```python
from build123d import *

# Parameters (mm, degrees)
F0_W     = 20
F0_H     = 95
F1_DEPTH = 6
F3_R     = 3
F5_R     = 4.25
F5_R_2   = 3
F6_DEPTH = 10


with BuildPart() as f1:
    # F0 (on Top) → F1 (new body, symmetric)
    with BuildSketch(Plane.XY):
        with Locations((10, 47.5)):
            Rectangle(F0_W, F0_H)
    extrude(amount=F1_DEPTH, both=True)

    # F4: sweep along a path in F2
    with BuildLine(Plane.XY) as f4_path:
        Line((13, 0), (13, 80))
        ThreePointArc((13, 80), (10.6568542495, 85.6568542495), (5, 88))
        Line((5, 88), (0, 88))
    # F3 (on face) → F4 (sweep, cut)
    with BuildSketch(Plane.XZ):
        with Locations((13, 0)):
            Circle(F3_R)
    sweep(path=f4_path.line, mode=Mode.SUBTRACT)

    # F5 (on face) → F6 (join)
    with BuildSketch(Plane.XZ):
        with Locations((13, 0)):
            Circle(F5_R)
        with Locations((13, 0)):
            Circle(F5_R_2, mode=Mode.SUBTRACT)
    extrude(amount=F6_DEPTH)

    # F7: F1 across face


with BuildPart() as f1_1:
    add(f1.part)
    add(f1.part.mirror(Plane(origin=(0, 46.4699702389, 0), x_dir=(0, -1, 0), z_dir=(-1, 0, 0))))


solid = f1_1.part
```
Part model, mm, in its own coordinate system. A direction names the side the tool comes from. Give positions to 0.01 mm unless a question says otherwise; leave off trailing zeros. Write each loop counter-clockwise with the first axis right and the second up, starting at its lowest first coordinate (ties: lowest second). Pieces come first, ordered by that corner, then holes. Notation, with made-up numbers: (48, 58.5) -> (69, 58.5) arc R17 cw to (69, 74.5) -> close; hole circle Ø11 at (-35.75, 11.25). An arc over 180 degrees is marked (long way). Put each result on its own line as item: value. Start each with the question number.
Item 1: Which spindle directions (+Z, -Z, +X, -X, +Y, -Y) get a long thin tool onto all of the face, cutting with end or side? Do faces 4 (the face through (20, 47, 0)), 5 (the face through (-10, 36, 0)). Say none if no direction does.
Item 2: Cut at A-A (z = 0). List the corners of the cut face in (x, y).
Item 3: Pin check, flat tips, straight feed: pin 1 Ø1 at (x, z) = (9, -4) entering from -Y; pin 2 Ø5 at (x, z) = (-13, 1) entering from -Y. Stop position of each tip, or through.
Item 4: Cut at D-D (y = 82). State how many separate pieces and enclosed holes the cut face has, then the cut area to 3 significant figures.
Item 5: Wall check: L1, parallel to X at y = 49.5, z = 0; L2, parallel to Z at x = -1.8, y = 88; L3, parallel to X at y = 72, z = 2. Give the ranges that are in metal, low to high. Write a range as [from, to].
Item 6: Pull direction X, two halves, no side cores. Call faces 1 (the face through (-20, 47, 0)), 2 (the face through (0, 0, 0)), 3 (the face through (0, 48, 6)): pulls with the +X half, pulls with the -X half, needs draft (parallel to the pull), parting line crosses it, or undercut.
Item 7: Cut at B-B (x = -3). List the corners of the cut face in (y, z).
Item 8: Cut at C-C (y = 42.5). List the corners of the cut face in (x, z), then the cut area to 3 significant figures.
Answer list:
1. face 4: +Z, -Z, +X, +Y, -Y
1. face 5: -Y
2. outline: (-20, 0) -> (-17.25, 0) -> (-17.25, -10) -> (-16, -10) -> (-16, 80) arc R11 cw to (-5, 91) -> (5, 91) arc R11 cw to (16, 80) -> (16, -10) -> (17.25, -10) -> (17.25, 0) -> (20, 0) -> (20, 95) -> (-20, 95) -> close; (-10, -10) -> (-8.75, -10) -> (-8.75, 0) -> (8.75, 0) -> (8.75, -10) -> (10, -10) -> (10, 80) arc R5 ccw to (5, 85) -> (-5, 85) arc R5 ccw to (-10, 80) -> close
3. pin 1: stops at y = 0
3. pin 2: stops at y = -10
4. separate pieces: 1
4. enclosed holes: 2
4. area: 421 mm2
5. L1: x = [-20, -16], [-10, 10], [16, 20]
5. L2: z = [-6, -3], [3, 6]
5. L3: x = [-20, -15.24], [-10.76, 10.76], [15.24, 20]
6. face 1: pulls with the -X half
6. face 2: undercut
6. face 3: needs draft
7. outline: (0, -6) -> (95, -6) -> (95, 6) -> (0, 6) -> close; hole circle Ø6 at (88, 0)
8. outline: (-20, -6) -> (20, -6) -> (20, 6) -> (-20, 6) -> close; hole circle Ø6 at (-13, 0); hole circle Ø6 at (13, 0)
8. area: 423 mm2
